Autodesk Inventor part; units mm, degrees
ref_plane "YZ Plane" through (0, 0, 0) normal (1, 0, 0) x (0, 1, 0)
ref_plane "XZ Plane" through (0, 0, 0) normal (0, 1, 0) x (-1, 0, 0)
ref_plane "XY Plane" through (0, 0, 0) normal (0, 0, 1) x (1, 0, 0)
sketch "Sketch1" plane through (0, 0, 0) normal (0, 0, 1) x (1, 0, 0)
  circle A0 centre (-9, 3.5) radius 1.5
  circle A1 centre (-2.5, 3.5) radius 1.5
  line L0 (0, 0) -> (-11.5, 0)
  line L1 (0, 5) -> (0, 0)
  arc A2 (0, 5) -> (-2, 7) centre (-2, 5) ccw
  line L2 (-11.5, 7) -> (-2, 7)
  line L3 (-11.5, 0) -> (-11.5, 7)
extrude "Extrusion1" add sketch "Sketch1" along normal blind 6
properties part number "yCarMid_c"
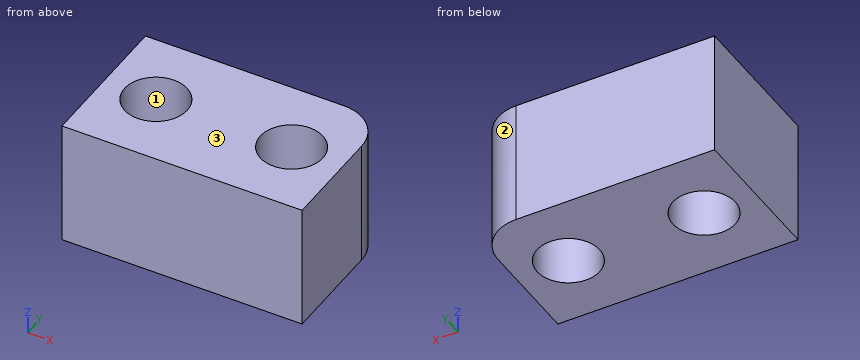
Geometry: final body of the model. Coordinates: model frame, mm. Face numbers are marked on the shaded views. Round coordinates to 2 decimals unless told otherwise and drop trailing zeros. Loops run counter-clockwise (first coordinate to the right, second up) from the corner with the lowest first, then second, coordinate; pieces in that order, holes last.
Q1. Pull-direction query (X, two-part tool) for the marked faces 1, 2 and 3; classes: released by +X, released by -X, zero draft, split by the parting line, or undercut.
Q2. Pin query (flat end, axial travel): P1, Ø2.5, axis at x = -9, y = 3.5, coming from the +Z side. Return the tip coordinate at first contact, or that it passes through.
Q3. Section A-A on z = 3.9. Return loops of the section in (x, y).
Q4. Material intervals for L1, parallel to Y at x = -9, z = 3.9; L2, parallel to X at y = 2.75, z = 3.15; L3, parallel to Y at x = -1.5, z = 1.4, sorted ascending.
Q5. Section C-C on x = -9. Return loops of the section in (y, z), plus the area to 3 significant figures.
Q6. Section D-D on y = 4.5. Return loops of the section in (x, z), plus the area to 3 significant figures.
Q7. Section B-B on y = 3.5. Return loops of the section in (x, z), plus the area to 3 significant figures.
Evaluation:
1. face 1: undercut
1. face 2: released by +X
1. face 3: zero draft
2. P1: passes through
3. outline: (-11.5, 0) - (0, 0) - (0, 5) arc R2 ccw to (-2, 7) - (-11.5, 7) - close; hole circle Ø3 at (-9, 3.5); hole circle Ø3 at (-2.5, 3.5)
4. L1: y = 0 to 2, 5 to 7
4. L2: x = -11.5 to -10.3, -7.7 to -3.8, -1.2 to 0
4. L3: y = 0 to 2.38, 4.62 to 6.94
5. outline: (0, 0) - (2, 0) - (2, 6) - (0, 6) - close; (5, 0) - (7, 0) - (7, 6) - (5, 6) - close
5. area: 24.0 mm2
6. outline: (-11.5, 0) - (-10.12, 0) - (-10.12, 6) - (-11.5, 6) - close; (-7.88, 0) - (-3.62, 0) - (-3.62, 6) - (-7.88, 6) - close; (-1.38, 0) - (0, 0) - (0, 6) - (-1.38, 6) - close
6. area: 42.2 mm2
7. outline: (-11.5, 0) - (-10.5, 0) - (-10.5, 6) - (-11.5, 6) - close; (-7.5, 0) - (-4, 0) - (-4, 6) - (-7.5, 6) - close; (-1, 0) - (0, 0) - (0, 6) - (-1, 6) - close
7. area: 33.0 mm2
